from build123d import *

# Parameters (mm, degrees)
EXTRUDE_359_DEPTH   = 5.3
SKETCH_4_W          = 0.6
SKETCH_4_H          = 11.005553499
CHAMFER_1890_SIZE   = 1
FILLET_1935_R       = 0.4
SKETCH_7_R          = 6.006178493
CUT_EXTRUDE_1_DEPTH = 10


with BuildPart() as part:
    # 草图1 → Extrude 359 (new body)
    with BuildSketch(Plane(origin=(0, 0, 0), x_dir=(0, 0, -1), z_dir=(1, 0, 0))):
        Polygon((6.5, 3.75277675), (6.5, -3.75277675), (0, -7.505553499), (-6.5, -3.75277675), (-6.5, 3.75277675), (0, 7.505553499), align=None)
    extrude(amount=EXTRUDE_359_DEPTH)

    # 草图2 → 凸台-旋转1 (revolve)
    with BuildSketch(Plane.XY, mode=Mode.PRIVATE) as revolve_1_sk:
        Polygon((0, 0), (45.3, 0), (45.3, 2.9175), (45.3, 4), (0, 4), align=None)
    revolve(revolve_1_sk.sketch.rotate(Axis((0, 0, 0), (1, 0, 0)), 90), axis=Axis((0, 0, 0), (1, 0, 0)))

    # 草图3 → 切除-旋转1 (revolve, cut)
    with BuildSketch(Plane.XY):
        Polygon((0, 6.5), (3.46730793, 12.505553499), (3.46730793, 17.505553499), (-10, 17.505553499), (-10, 6.5), align=None)
    revolve(axis=Axis((0, 0, 0), (1, 0, 0)), mode=Mode.SUBTRACT)

    # 草图5 → 切除-旋转2 (revolve, cut)
    with BuildSketch(Plane.XY):
        Polygon((5.3, 6.5), (1.83269207, 12.505553499), (1.83269207, 17.505553499), (11.83269207, 17.505553499), (11.83269207, 6.5), align=None)
    revolve(axis=Axis((0, 0, 0), (1, 0, 0)), mode=Mode.SUBTRACT)

    # 草图4 → 切除-旋转3 (revolve, cut)
    with BuildSketch(Plane.XY, mode=Mode.PRIVATE) as cut_revolve_3_sk:
        with Locations((5, 12.00277675)):
            Rectangle(SKETCH_4_W, SKETCH_4_H)
    revolve(cut_revolve_3_sk.sketch.rotate(Axis((0, 0, 0), (1, 0, 0)), 270), axis=Axis((0, 0, 0), (1, 0, 0)), mode=Mode.SUBTRACT)

    # Chamfer 1890
    chamfer_1890_edges = [part.edges().sort_by_distance(p)[0] for p in [
        (45.3, 0, -4),
    ]]
    chamfer(chamfer_1890_edges, length=CHAMFER_1890_SIZE)

    # Fillet 1935
    fillet_1935_edges = [part.edges().sort_by_distance(p)[0] for p in [
        (5.3, 0, -4),
    ]]
    fillet(fillet_1935_edges, radius=FILLET_1935_R)

    # 草图7 → 切除-拉伸1 (cut)
    with BuildSketch(Plane(origin=(45.3, 0, 0), x_dir=(0, 0, -1), z_dir=(1, 0, 0))):
        Circle(SKETCH_7_R)
    extrude(amount=-CUT_EXTRUDE_1_DEPTH, mode=Mode.SUBTRACT)


solid = part.part
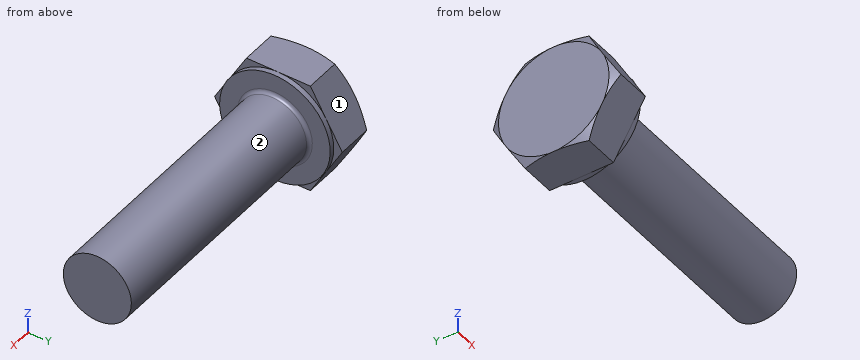
Here's how the part is built. I have some questions about the finished solid (model axes, mm). Face numbers are marked on the shaded views. A direction names the side the tool comes from. Coordinates: 2 decimals unless noted, no trailing zeros. Write each loop counter-clockwise with the first axis right and the second up, starting at its lowest first coordinate (ties: lowest second). Pieces come first, ordered by that corner, then holes.
Item 1: If I drill on line 1 (X direction, y = 2.25, z = 4.25); line 2 (Y direction, x = 30, z = -2.25); line 3 (Y direction, x = 5, z = -5.25), over which ranges is the centre line in solid material (lowest first)?
Item 2: I want a section at B-B on x = 15.5. Write out the boundary of the cut face in (y, z), and give its area (3 significant figures).
Item 3: Will these pins go through, and if not, where does the flat tip stop? pin 1 (1 mm diameter, centred on y = -1.5, z = -5, fed in from +X); pin 2 (1 mm diameter, centred on y = -1, z = -2.5, fed in from -X); pin 3 (4 mm diameter, centred on x = 6, y = -5.5, fed in from -Z); pin 4 (1 mm diameter, centred on x = 30, y = 3.5, fed in from -Z).
Item 4: I want a section at A-A on x = 3. Write out the boundary of the cut face in (y, z), and give its area (3 significant figures).
Item 5: On a 3-axis mill with a long thin cutter (end or side, diameter ignored), from which of +Z, -Z, +X, -X, +Y, -Y can I reach the whole of each face in a straight line? I mean the marked faces 1 and 2. Say none if no direction works.
Findings below:
1. line 1: x = 0 to 5.3
1. line 2: y = -3.31 to 3.31
1. line 3: y = -3.83 to 3.83
2. outline: circle Ø8 at (0, 0)
2. area: 50.3 mm2
3. pin 1: stops at x = 5.3
3. pin 2: stops at x = 0
3. pin 3: stops at z = -6.11
3. pin 4: stops at z = -2.65
4. outline: (-7.51, 0) - (-3.75, -6.5) - (3.75, -6.5) - (7.51, 0) - (3.75, 6.5) - (-3.75, 6.5) - close
4. area: 146 mm2
5. face 1: +Z, +X, -X, +Y
5. face 2: +X
